```python
from build123d import *
from OCP.BRepFilletAPI import BRepFilletAPI_MakeChamfer

# Parameters (mm, degrees)
SZKIC1_W                    = 7.1
SZKIC1_H                    = 5.9
DODANIE_WYCI_GNI_CIE1_DEPTH = 2.4
SFAZOWANIE1_SIZE            = 1.1
SFAZOWANIE1_SIZE2           = 0.1
SFAZOWANIE2_SIZE            = 0.1
SFAZOWANIE2_SIZE2           = 1.1
SZKIC2_W                    = 0.9
SZKIC2_H                    = 5.7
DODANIE_WYCI_GNI_CIE2_DEPTH = 0.001
SZKIC3_W                    = 0.15
SZKIC3_H                    = 5.9
WYTNIJ_WYCI_GNI_CIE1_DEPTH  = 1.15
SFAZOWANIE3_SIZE            = 0.15
SZKIC4_W                    = 0.2
SZKIC4_H                    = 3
SFAZOWANIE3_OF_LUSTRO1_SIZE = 0.15


with BuildPart() as part:
    # Szkic1 → Dodanie-wyciągnięcie1 (new body)
    with BuildSketch(Plane.XY):
        Rectangle(SZKIC1_W, SZKIC1_H)
    extrude(amount=DODANIE_WYCI_GNI_CIE1_DEPTH)

    # Sfazowanie1: one chamfer whose edges measure the first distance from different faces: ONE call of the kernel's chamfer builder (chamfer() names one face for all edges)
    sfazowanie1_edges_1 = [part.edges().sort_by_distance(p)[0] for p in [
        (3.55, 0, 2.4),
    ]]
    sfazowanie1_side_1 = [part.faces().sort_by_distance(p)[0] for p in [
        (3.55, 0, 1.2),
    ]]
    sfazowanie1_edges_2 = [part.edges().sort_by_distance(p)[0] for p in [
        (0, 2.95, 2.4),
    ]]
    sfazowanie1_side_2 = [part.faces().sort_by_distance(p)[0] for p in [
        (0, 2.95, 1.2),
    ]]
    sfazowanie1_edges_3 = [part.edges().sort_by_distance(p)[0] for p in [
        (-3.55, 0, 2.4),
    ]]
    sfazowanie1_side_3 = [part.faces().sort_by_distance(p)[0] for p in [
        (-3.55, 0, 1.2),
    ]]
    sfazowanie1_edges_4 = [part.edges().sort_by_distance(p)[0] for p in [
        (0, -2.95, 2.4),
    ]]
    sfazowanie1_side_4 = [part.faces().sort_by_distance(p)[0] for p in [
        (0, -2.95, 1.2),
    ]]
    sfazowanie1 = BRepFilletAPI_MakeChamfer(part.part.solid().wrapped)
    for e in sfazowanie1_edges_1:
        sfazowanie1.Add(SFAZOWANIE1_SIZE, SFAZOWANIE1_SIZE2, e.wrapped, sfazowanie1_side_1[0].wrapped)  # the first distance lies on this face
    for e in sfazowanie1_edges_2:
        sfazowanie1.Add(SFAZOWANIE1_SIZE, SFAZOWANIE1_SIZE2, e.wrapped, sfazowanie1_side_2[0].wrapped)  # the first distance lies on this face
    for e in sfazowanie1_edges_3:
        sfazowanie1.Add(SFAZOWANIE1_SIZE, SFAZOWANIE1_SIZE2, e.wrapped, sfazowanie1_side_3[0].wrapped)  # the first distance lies on this face
    for e in sfazowanie1_edges_4:
        sfazowanie1.Add(SFAZOWANIE1_SIZE, SFAZOWANIE1_SIZE2, e.wrapped, sfazowanie1_side_4[0].wrapped)  # the first distance lies on this face
    add(Compound.cast(sfazowanie1.Shape()), mode=Mode.REPLACE)

    # Sfazowanie2
    sfazowanie2_edges = [part.edges().sort_by_distance(p)[0] for p in [
        (0, 2.95, 0),
        (3.55, 0, 0),
        (0, -2.95, 0),
        (-3.55, 0, 0),
    ]]
    sfazowanie2_side = [part.faces().sort_by_distance(p)[0] for p in [
        (0, 0, 0),
    ]]
    chamfer(sfazowanie2_edges, length=SFAZOWANIE2_SIZE, length2=SFAZOWANIE2_SIZE2, reference=sfazowanie2_side[0])

    # Szkic2 → Dodanie-wyciągnięcie2 (add)
    with BuildSketch(Plane.XY.offset(2.4)):
        with Locations((-2.5, 0)):
            Rectangle(SZKIC2_W, SZKIC2_H)
    extrude(amount=DODANIE_WYCI_GNI_CIE2_DEPTH)

    # Szkic3 → Wytnij-wyciągnięcie1 (cut)
    with BuildSketch(Plane.ZY.offset(3.55)):
        with Locations((0.075, 0)):
            Rectangle(SZKIC3_W, SZKIC3_H)
    wytnij_wyci_gni_cie1 = extrude(amount=-WYTNIJ_WYCI_GNI_CIE1_DEPTH, mode=Mode.SUBTRACT)

    # Sfazowanie3
    sfazowanie3_edges = [part.edges().sort_by_distance(p)[0] for p in [
        (-2.4, 0, 0),
    ]]
    chamfer(sfazowanie3_edges, length=SFAZOWANIE3_SIZE - 0.0001)  # a hair under: the kernel refuses the full size

    # Wyciągnięcie po ścieżce1: sweep along a path in Szkic5
    with BuildLine(Plane(origin=(0, 0, 0), x_dir=(1, 0, 0), z_dir=(0, 1, 0))) as wyci_gni_cie_po_cie_ce1_path:
        Line((-3.55, -1.3), (-3.65, -1.3))
        ThreePointArc((-3.65, -1.3), (-3.826776695, -1.226776695), (-3.9, -1.05))
        Line((-3.9, -1.05), (-3.9, -0.2))
        ThreePointArc((-3.9, -0.2), (-3.826776695, -0.023223305), (-3.65, 0.05))
        Line((-3.65, 0.05), (-2.7, 0.05))
    # Szkic4 → Wyciągnięcie po ścieżce1 (sweep)
    with BuildSketch(Plane.ZY.offset(3.55)):
        with Locations((1.2, 0)):
            Rectangle(SZKIC4_W, SZKIC4_H)
    wyci_gni_cie_po_cie_ce1 = sweep(path=wyci_gni_cie_po_cie_ce1_path.line)

    # Lustro1: Wytnij-wyciągnięcie1, Wyciągnięcie po ścieżce1 across plane
    add(wytnij_wyci_gni_cie1.mirror(Plane(origin=(0, 0, 0), x_dir=(0, 0, 1), z_dir=(1, 0, 0))), mode=Mode.SUBTRACT)
    add(wyci_gni_cie_po_cie_ce1.mirror(Plane(origin=(0, 0, 0), x_dir=(0, 0, 1), z_dir=(1, 0, 0))))

    # Sfazowanie3 of Lustro1
    sfazowanie3_of_lustro1_edges = [part.edges().sort_by_distance(p)[0] for p in [
        (2.4, 0, 0),
    ]]
    chamfer(sfazowanie3_of_lustro1_edges, length=SFAZOWANIE3_OF_LUSTRO1_SIZE - 0.0001)  # a hair under: the kernel refuses the full size


solid = part.part
```
Could you check a few things on this model? Use its own coordinates, in mm. A direction names the side the tool comes from. Give positions to 0.01 mm unless a question says otherwise; leave off trailing zeros. Loops run counter-clockwise (first coordinate to the right, second up) from the corner with the lowest first, then second, coordinate; pieces in that order, holes last. Notation, with made-up numbers: (21.5, 18) -> (73.5, 18) arc R9 ccw to (73.5, 33) -> close; hole circle Ø8 at (25, 62.5). An arc over 180 degrees is marked (long way). Put each result on its own line as item: value.
(1) Imagine slicing it at A-A on z = 0.85. Write out the boundary of the cut face in (x, y).
Computed:
outline: (-3.9, -1.5) -> (-3.7, -1.5) -> (-3.7, 1.5) -> (-3.9, 1.5) -> close; (-3.53, -2.93) -> (3.53, -2.93) -> (3.53, 2.93) -> (-3.53, 2.93) -> close; (3.7, -1.5) -> (3.9, -1.5) -> (3.9, 1.5) -> (3.7, 1.5) -> close
(2) Thinking about a two-plate mould opening in X: for faces 1 (the face through (-3.7, 0, 0.6)), 2 (the face through (-3.5, -0.04, 1.86)), 3 (the face through (-0.05, 2.9, 0.56)), 4 (the face through (3.507, -0.041, 0.632)), which applies, pulls with the +X half, pulls with the -X half, needs draft (parallel to the pull), parting line crosses it, or undercut?
Computed:
face 1: undercut
face 2: pulls with the -X half
face 3: needs draft
face 4: undercut
(3) For faces 5 (the face through (0, 0, 0)), 6 (the face through (3.9, 0, 0.6)), 7 (the face through (-3.507, -0.041, 0.632)), which set-ups out of +Z, -Z, +X, -X, +Y, -Y let a thin tool reach every point of the face, with its end or its side?
Computed:
face 5: -Z, +Y, -Y
face 6: +Z, -Z, +X, +Y, -Y
face 7: +Y, -Y
(4) Please list where these lines run through material, in increasing order: probe 1 along X at (y, z) = (0.15, 0.25); probe 2 along Z at (x, y) = (-3, 2.65); probe 3 along Z at (x, y) = (1.75, -0.7). Write a range as [from, to].
Computed:
probe 1: [-3.9, -3.7], [-3.47, 3.47], [3.7, 3.9]
probe 2: [0.15, 2.4]
probe 3: [0, 2.4]
(5) Imagine slicing it at D-D on y = -0.7. State how many separate pieces and enclosed holes the cut face has, plus the area to 3 significant figures.
Computed:
separate pieces: 1
enclosed holes: 2
area: 17.4 mm^2
